Source: CAD feature listing. Evaluate the final solid. Frame: model axes, mm. Face numbers are marked on the shaded views. A direction names the side the tool comes from. Give positions to 0.01 mm unless a question says otherwise; leave off trailing zeros. Order: outer loops, then holes, each group sorted by start corner. A loop starts at its lowest first (then second) coordinate and runs counter-clockwise, first axis right, second up. Notation, with made-up numbers: M 66,67 L 107,67 A27 ccw 107,102 Z; hole C 21,29.25 d3. An arc over 180 degrees is marked long. Use CSV: the item, a comma, the result in double quotes. Start each with the question number.
1. Section query B-B, the plane z = -6. Return the cut outline in (x, y).
2. Section query A-A, the plane y = 28. Return the cut outline in (x, z), plus the area to 3 significant figures.
3. Pin query (flat end, axial travel): P1, Ø3, axis at x = 1, z = 12, coming from the -Y side; P2, Ø1.2, axis at x = -10.5, y = 24.5, coming from the -Z side; P3, Ø3, axis at x = 8.5, z = 12, coming from the +Y side. Return the tip coordinate at first contact, or that it passes through.
4. Section query D-D, the plane y = 22.25. Return the cut outline in (x, z), plus the area to 3 significant figures.
5. Line query: line 1 along X through (y, z) = (23.45, 0); line 2 along Z through (x, y) = (-17, 28); line 3 along X through (y, z) = (22.75, -11.5). Output: solid intervals per line, ascending. Write a range as [from, to].
6. Reachability of the marked faces 1, 2, 3, 4 and 5 from +Z, -Z, +X, -X, +Y, -Y: full face, straight path, thin tool, end or side. Return the list, or none.
7. Section query C-C, the plane x = -9. Return the cut outline in (y, z).
8. Mould query, pull axis X, two halves, no side actions, for the marked faces 6, 7 and 8. Classes: released by +X, released by -X, zero draft, split by the parting line, or undercut.
from build123d import *

# Parameters (mm, degrees)
SERVO_SHELF_START                = 21.4
SERVO_SHELF_PROFILE_W            = 46
SERVO_SHELF_PROFILE_H            = 36
SERVO_SHELF_DEPTH                = 4
REAR_CLAMPING_BLOCK_START        = -18
REAR_CLAMPING_BLOCK_PROFILE_W    = 7
REAR_CLAMPING_BLOCK_PROFILE_H    = 10
REAR_CLAMPING_BLOCK_DEPTH        = 36
SERVO_BODY_WINDOW_START          = 20.4
SERVO_BODY_WINDOW_PROFILE_W      = 23.8
SERVO_BODY_WINDOW_PROFILE_H      = 13
SERVO_BODY_WINDOW_DEPTH          = 25.744213361
YAW_SERVO_M2_FASTENERS_START     = 20.4
YAW_SERVO_M2_FASTENERS_PROFILE_R = 1.3
YAW_SERVO_M2_FASTENERS_DEPTH     = 25.744213361
LEFT_NUT_ACCESS_START            = 20
LEFT_NUT_ACCESS_PROFILE_W        = 10
LEFT_NUT_ACCESS_PROFILE_H        = 8
LEFT_NUT_ACCESS_DEPTH            = 26.144213361
RIGHT_NUT_ACCESS_START           = 20
RIGHT_NUT_ACCESS_PROFILE_W       = 10
RIGHT_NUT_ACCESS_PROFILE_H       = 8
RIGHT_NUT_ACCESS_DEPTH           = 26.144213361
REAR_CLAMPING_M3_HOLES_START     = -25
REAR_CLAMPING_M3_PROFILE_R       = 1.6
REAR_CLAMPING_M3_HOLES_DEPTH     = 11
FILLET1_R                        = 3
FILLET2_R                        = 1
BOSS_EXTRUDE1_START              = -36
BOSS_EXTRUDE1_DEPTH              = 36


with BuildPart() as part:
    # Servo_shelf_profile → Servo_shelf (new body)
    with BuildSketch(Plane(origin=(0, 0, 0), x_dir=(1, 0, 0), z_dir=(0, 1, 0)).offset(SERVO_SHELF_START)):
        with Locations((2, 0)):
            Rectangle(SERVO_SHELF_PROFILE_W, SERVO_SHELF_PROFILE_H)
    extrude(amount=SERVO_SHELF_DEPTH)

    # Rear_clamping_block_profile → Rear_clamping_block (add)
    with BuildSketch(Plane.XY.offset(REAR_CLAMPING_BLOCK_START)):
        with Locations((-17.5, 28)):
            Rectangle(REAR_CLAMPING_BLOCK_PROFILE_W, REAR_CLAMPING_BLOCK_PROFILE_H)
    extrude(amount=REAR_CLAMPING_BLOCK_DEPTH)

    # Servo_body_window_profile → Servo_body_window (cut, through all)
    with BuildSketch(Plane(origin=(0, 0, 0), x_dir=(1, 0, 0), z_dir=(0, 1, 0)).offset(SERVO_BODY_WINDOW_START)):
        with Locations((5.5, 0)):
            Rectangle(SERVO_BODY_WINDOW_PROFILE_W, SERVO_BODY_WINDOW_PROFILE_H)
    extrude(amount=SERVO_BODY_WINDOW_DEPTH, mode=Mode.SUBTRACT)

    # Yaw_servo_M2_fasteners_profile → Yaw_servo_M2_fasteners (cut, through all)
    with BuildSketch(Plane(origin=(0, 0, 0), x_dir=(1, 0, 0), z_dir=(0, 1, 0)).offset(YAW_SERVO_M2_FASTENERS_START)):
        with Locations(Location((-9, 0, 0), (0, 0, 90))):
            Circle(YAW_SERVO_M2_FASTENERS_PROFILE_R)
        with Locations(Location((20, 0, 0), (0, 0, 90))):
            Circle(YAW_SERVO_M2_FASTENERS_PROFILE_R)
    extrude(amount=YAW_SERVO_M2_FASTENERS_DEPTH, mode=Mode.SUBTRACT)

    # Left_nut_access_profile → Left_nut_access (cut, through all)
    with BuildSketch(Plane(origin=(0, 0, 0), x_dir=(1, 0, 0), z_dir=(0, 1, 0)).offset(LEFT_NUT_ACCESS_START)):
        with Locations((-9, 12)):
            Rectangle(LEFT_NUT_ACCESS_PROFILE_W, LEFT_NUT_ACCESS_PROFILE_H)
    extrude(amount=LEFT_NUT_ACCESS_DEPTH, mode=Mode.SUBTRACT)

    # Right_nut_access_profile → Right_nut_access (cut, through all)
    with BuildSketch(Plane(origin=(0, 0, 0), x_dir=(1, 0, 0), z_dir=(0, 1, 0)).offset(RIGHT_NUT_ACCESS_START)):
        with Locations((-9, -12)):
            Rectangle(RIGHT_NUT_ACCESS_PROFILE_W, RIGHT_NUT_ACCESS_PROFILE_H)
    extrude(amount=RIGHT_NUT_ACCESS_DEPTH, mode=Mode.SUBTRACT)

    # Rear_clamping_M3_profile → Rear_clamping_M3_holes (cut)
    with BuildSketch(Plane(origin=(0, 0, 0), x_dir=(0, 0, -1), z_dir=(1, 0, 0)).offset(REAR_CLAMPING_M3_HOLES_START)):
        with Locations((12, 28)):
            Circle(REAR_CLAMPING_M3_PROFILE_R)
        with Locations((-12, 28)):
            Circle(REAR_CLAMPING_M3_PROFILE_R)
    extrude(amount=REAR_CLAMPING_M3_HOLES_DEPTH, mode=Mode.SUBTRACT)

    # Fillet1
    fillet1_edges = [part.edges().sort_by_distance(p)[0] for p in [
        (-4, 23.4, 16),
        (-4, 23.4, 8),
        (-4, 23.4, -8),
        (-4, 23.4, -16),
    ]]
    fillet(fillet1_edges, radius=FILLET1_R)

    # Fillet2
    fillet2_edges = [part.edges().sort_by_distance(p)[0] for p in [
        (-14, 23.4, 16),
        (5.5, 25.4, 18),
        (-14, 25.4, 17),
        (5.5, 25.4, -18),
        (-14, 29.2, 18),
        (-14, 29.2, -18),
        (-14, 25.4, -17),
        (-14, 23.4, -16),
    ]]
    fillet(fillet2_edges, radius=FILLET2_R)

    # Sketch1 → Boss-Extrude1 (add)
    with BuildSketch(Plane(origin=(0, 0, -18), x_dir=(-1, 0, 0), z_dir=(0, 0, -1)).offset(BOSS_EXTRUDE1_START)):
        Polygon((14, 21.4), (21, 15), (21, 21.4), align=None)
    extrude(amount=BOSS_EXTRUDE1_DEPTH)


solid = part.part
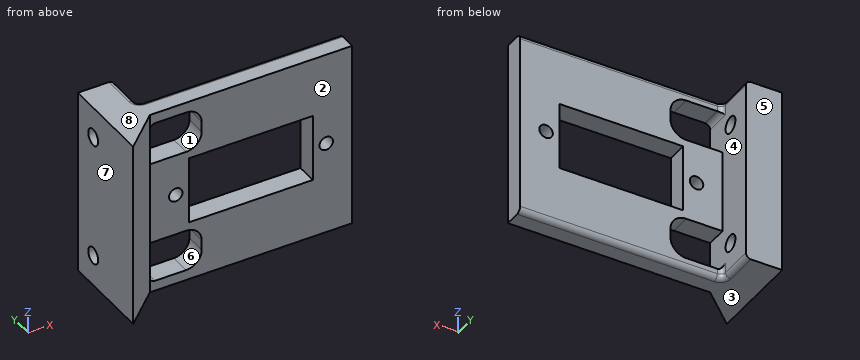
Result set:
1,outline,"M -21,15 L -14,21.4 L -6.4,21.4 L -6.4,25.4 L -14,25.4 L -14,33 L -21,33 Z; M 17.4,21.4 L 25,21.4 L 25,25.4 L 17.4,25.4 Z"
2,outline,"M -21,-18 L -15,-18 A1 ccw -14,-17 L -14,-13.6 L -21,-13.6 Z; M -21,-10.4 L -14,-10.4 L -14,10.4 L -21,10.4 Z; M -21,13.6 L -14,13.6 L -14,17 A1 ccw -15,18 L -21,18 Z"
2,area,"207 mm2"
3,P1,"y = 21.4"
3,P2,"z = -18"
3,P3,"y = 25.4"
4,outline,"M -21,-18 L 25,-18 L 25,18 L -21,18 Z; hole M -14,-15 A1 ccw -13,-16 L -7,-16 A3 ccw -4,-13 L -4,-11 A3 ccw -7,-8 L -14,-8 Z; hole M -14,8 L -7,8 A3 ccw -4,11 L -4,13 A3 ccw -7,16 L -13,16 A1 ccw -14,15 Z; hole C -9,0 d2.6; hole M -6.4,-6.5 L 17.4,-6.5 L 17.4,6.5 L -6.4,6.5 Z; hole C 20,0 d2.6"
4,area,"1,180 mm2"
5,line 1,"[-21, -10.3], [-7.7, -6.4], [17.4, 18.7], [21.3, 25]"
5,line 2,"[-18, -13.6], [-10.4, 10.4], [13.6, 18]"
5,line 3,"[-21, -14], [-4, 25]"
6,face 1,"+Y, -Y"
6,face 2,"+Z, -Z, +X, -Y"
6,face 3,"-Z, +X, -X, +Y, -Y"
6,face 4,"+Y"
6,face 5,"+Z, -Z, +X, -X, +Y"
7,outline,"M 21.4,-18 L 24.4,-18 A1 ccw 25.4,-17 L 25.4,-16 L 21.4,-16 Z; M 21.4,-8 L 25.4,-8 L 25.4,-1.3 L 21.4,-1.3 Z; M 21.4,1.3 L 25.4,1.3 L 25.4,8 L 21.4,8 Z; M 21.4,16 L 25.4,16 L 25.4,17 A1 ccw 24.4,18 L 21.4,18 Z"
8,face 6,"undercut"
8,face 7,"released by -X"
8,face 8,"zero draft"
